Autodesk Inventor part; units mm, degrees
ref_plane "YZ Plane" through (0, 0, 0) normal (1, 0, 0) x (0, 1, 0)
ref_plane "XZ Plane" through (0, 0, 0) normal (0, 1, 0) x (-1, 0, 0)
ref_plane "XY Plane" through (0, 0, 0) normal (0, 0, 1) x (1, 0, 0)
sketch "Sketch1" plane through (0, 0, 0) normal (0, 0, 1) x (1, 0, 0)
  line L0 (0, 0) -> (6.3089, 0)
  line L1 (0, 0) -> (0, 8.1845)
  line L2 (4.5, 24) -> (4.5, -35)
  line L3 (4.5, -35) -> (-4.5, -35)
  line L4 (-4.5, -35) -> (-4.5, 24)
  line L5 (-6.35, 35) -> (6.35, 35)
  line L6 (6.35, 35) -> (6.35, 24)
  line L7 (-6.35, 24) -> (-6.35, 35)
  line L8 (6.35, 24) -> (4.5, 24)
  line L9 (-4.5, 24) -> (-6.35, 24)
  dimension "d4" = 9
  dimension "d5" = 12.7
  dimension "d6" = 70
  dimension "d7" = 11
extrude "Extrusion1" add sketch "Sketch1" along normal blind 0.5
sketch "Sketch2" plane through (-6.35, 34.5, 0) normal (0, 1, 0) x (-1, 0, 0)
  line L0 (-12.7, 0) -> (0, 0)
  line L1 (0, 0) -> (0, 4)
  line L2 (0, 4) -> (-12.7, 4)
  line L3 (-12.7, 4) -> (-12.7, 0)
edge flange "Flange1" height 4 angle 90 thickness 0.5 bend radius 0.5 thickness toward (0, 1, 0) relief straight relief width 0.5 relief depth 0.25 edges at (0, 35, 0.5) wall of the first edge with corners at (6.35, 34.5, 0) (-6.35, 34.5, 0) (-6.35, 34.5, 4) (6.35, 34.5, 4)
bend "Bend1"
corner "Corner1"
sketch "Sketch4" plane through (4.5, -34.5, 0) normal (0, -1, 0) x (1, 0, 0)
  line L0 (-9, 0) -> (0, 0)
  line L1 (0, 0) -> (0, 4)
  line L2 (0, 4) -> (-9, 4)
  line L3 (-9, 4) -> (-9, 0)
edge flange "Flange3" height 4 angle 90 thickness 0.5 bend radius 0.5 thickness toward (0, -1, 0) relief straight relief width 0.5 relief depth 0.25 edges at (0, -35, 0.5) wall of the first edge with corners at (-4.5, -34.5, 0) (4.5, -34.5, 0) (4.5, -34.5, 4) (-4.5, -34.5, 4)
bend "Bend3"
corner "Corner3"
equation "\"d8\" = BendReliefWidth"
equation "\"d9\" = BendReliefDepth"
equation "\"d10\" = MinimumRemnant"
equation "\"d11\" = BendRadius"
equation "\"d14\" = BendRadius"
equation "\"d15\" = CornerReliefSize"
equation "\"d16\" = GapSize"
equation "\"d17\" = JacobiRadiusSize"
equation "\"d28\" = BendReliefWidth"
equation "\"d29\" = BendReliefDepth"
equation "\"d30\" = MinimumRemnant"
equation "\"d31\" = BendRadius"
equation "\"d34\" = BendRadius"
equation "\"d35\" = CornerReliefSize"
equation "\"d36\" = GapSize"
equation "\"d37\" = JacobiRadiusSize"
equation "\"BendRadius\" = Thickness"
equation "\"BendReliefWidth\" = Thickness"
equation "\"BendReliefDepth\" = 0.5 * Thickness"
equation "\"CornerReliefSize\" = 4 * Thickness"
equation "\"MinimumRemnant\" = 2 * Thickness"
equation "\"TransitionRadius\" = BendRadius"
equation "\"JacobiRadiusSize\" = Thickness"
equation "\"GapSize\" = Thickness"
properties material "Aluminum-6061"
Can you work these out from the model? Positions are in its coordinate system, mm. A direction names the side the tool comes from. Give positions to 0.01 mm unless a question says otherwise; leave off trailing zeros. Write each loop counter-clockwise with the first axis right and the second up, starting at its lowest first coordinate (ties: lowest second). Pieces come first, ordered by that corner, then holes. Notation, with made-up numbers: (-15.5, 14) -> (-7.5, 14) arc R16 ccw to (-7.5, 20) -> close; hole circle Ø7 at (50, 43.5). An arc over 180 degrees is marked (long way). Answer as a JSON object with one key per item and string values. Group by question number.
Item 1: I'm going to push a flat-ended pin straight in: P1, Ø2, axis at y = -11.5, z = 2.5, coming from the -X side. Where does the tip first touch, or does it pass through?
Item 2: Suppose I cut it at B-B (x = -1.75). Please give me the cut outline in (y, z), plus the area to 3 significant figures.
Item 3: Please list where these lines run through material, in increasing order: line 1 (Y direction, x = 2.75, z = 1.15); line 2 (X direction, y = 16, z = 0.45); line 3 (Z direction, x = -4, y = -29.5). Write a range as [from, to].
Item 4: Suppose I cut it at A-A (z = 3.15). Please give me the cut outline in (x, y), plus the area to 4 significant figures.
Item 5: Suppose I cut it at C-C (y = -15.5). Please give me the cut outline in (x, z).
Item 6: Suppose I cut it at D-D (x = 5.5). Please give me the cut outline in (y, z), plus the area to 3 significant figures.
Item 7: For faces 1 (the face through (4.5, -5.6, 0.2)), 2 (the face through (0, 0, 0)), 3 (the face through (0, 34.5, 2)), which set-ups out of +Z, -Z, +X, -X, +Y, -Y let a thin tool reach every point of the face, with its end or its side?
Item 8: We'd pull the mould along Y, two halves only. Please class faces 4 (the face through (0, 0, 0.5)), 5 (the face through (0, -34.5, 2)), 6 (the face through (0, -35, 3)), 7 (the face through (-4.5, -5.6, 0.2)): +Y half, -Y half, draft (parallel to the pull), parting line (faces both ways), or undercut.
Findings:
{
 "1": {"P1": "passes through"},
 "2": {"outline": "(-35, 1) arc R1 ccw to (-34, 0) -> (34, 0) arc R1 ccw to (35, 1) -> (35, 4) -> (34.5, 4) -> (34.5, 1) arc R0.5 cw to (34, 0.5) -> (-34, 0.5) arc R0.5 cw to (-34.5, 1) -> (-34.5, 4) -> (-35, 4) -> close", "area": "38.2 mm²"},
 "3": {"line 1": "y = [-35, -34.5], [34.5, 35]", "line 2": "x = [-4.5, 4.5]", "line 3": "z = [0, 0.5]"},
 "4": {"outline": "(-6.35, 34.5) -> (6.35, 34.5) -> (6.35, 35) -> (-6.35, 35) -> close; (-4.5, -35) -> (4.5, -35) -> (4.5, -34.5) -> (-4.5, -34.5) -> close", "area": "10.85 mm²"},
 "5": {"outline": "(-4.5, 0) -> (4.5, 0) -> (4.5, 0.5) -> (-4.5, 0.5) -> close"},
 "6": {"outline": "(24, 0) -> (34, 0) arc R1 ccw to (35, 1) -> (35, 4) -> (34.5, 4) -> (34.5, 1) arc R0.5 cw to (34, 0.5) -> (24, 0.5) -> close", "area": "7.09 mm²"},
 "7": {"face 1": "+Z, -Z, +X, -Y", "face 2": "-Z, +X, -X, +Y, -Y", "face 3": "+Z, +X, -X"},
 "8": {"face 4": "undercut", "face 5": "undercut", "face 6": "-Y half", "face 7": "draft"}
}
